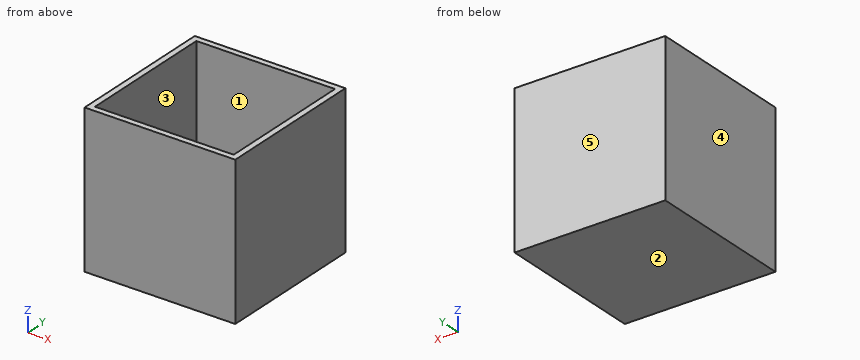
Autodesk Fusion 360 part; units mm, degrees
sketch "Sketch1" plane through (0, 0, 0) normal (0, 1, 0) x (1, 0, 0)
  line L0 (10, 10) -> (-10, 10)
  line L1 (-10, 10) -> (-10, -10)
  line L2 (-10, -10) -> (10, -10)
  line L3 (10, -10) -> (10, 10)
  line L4 (10, 10) -> (-10, -10) construction
  line L5 (-10, 10) -> (10, -10) construction
  dimension "d1" = 20
  dimension "d2" = 20
extrude "Extrude1" add sketch "Sketch1" along normal blind 20
sketch "Sketch2" plane through (0, 0, 10) normal (0, 0, 1) x (-1, 0, 0)
  line L0 (10, 0) -> (-10, 0)
  line L1 (-10, 0) -> (-10, -20)
  line L2 (-10, -20) -> (10, -20)
  line L3 (10, -20) -> (10, 0)
  line L4 (9.2, -0.8) -> (9.2, -19.2)
  line L5 (9.2, -19.2) -> (-9.2, -19.2)
  line L6 (-9.2, -19.2) -> (-9.2, -0.8)
  line L7 (-9.2, -0.8) -> (9.2, -0.8)
  dimension "d5" = 0.8
  dimension "d6" = 0.8
  dimension "d7" = 0.8
  dimension "d8" = 0.8
extrude "Extrude2" cut sketch "Sketch2" against normal blind 19.2 contours L4 L5 L6 L7
The model under review builds one solid part; all positions refer to its coordinate system, in mm. Face numbers are marked on the shaded views. A direction names the side the tool comes from. Give positions to 0.01 mm unless a question says otherwise; leave off trailing zeros. Write each loop counter-clockwise with the first axis right and the second up, starting at its lowest first coordinate (ties: lowest second). Pieces come first, ordered by that corner, then holes. Notation, with made-up numbers: M 22.5,-31 L 61.5,-31 A4 ccw 61.5,-25 Z; hole C -15.5,5 d2. An arc over 180 degrees is marked long. One line per question, with ' | ' between items. Start each with the question number.
Item 1: We need section C-C on y = 3. Write out the cut boundary in (x, z).
Item 2: We need section A-A on z = 3.5. Write out the cut boundary in (x, y), plus the area to 3 significant figures.
Item 3: Draft analysis for pull direction X (two halves, no side actions). For the marked faces 3, 4 and 5, state which applies: released by +X, released by -X, zero draft, split by the parting line, or undercut.
Item 4: For the marked faces 1 and 2, list the 3-axis set-ups (+Z, -Z, +X, -X, +Y, -Y) from which the entire face can be reached by the end or side of a thin tool; tool diameter is ignored.
Item 5: For pin 1 (9 mm diameter, centred on x = -3.5, y = 6.5, fed in from +Z), flat-tipped, find the tip position at first contact; note if it passes through.
Item 6: Wall thickness on line 1 (X direction, y = 2, z = -8.5); line 2 (Y direction, x = 7.75, z = 7.5); line 3 (Z direction, x = 7, y = 18): over which ranges is each line inside the solid? List them lowest first. Write a range as from..to.
Item 7: We need section B-B on x = 3. Write out the cut boundary in (y, z).
Results found:
1) outline: M -10,-10 L 10,-10 L 10,10 L 9.2,10 L 9.2,-9.2 L -9.2,-9.2 L -9.2,10 L -10,10 Z
2) outline: M -10,0 L 10,0 L 10,20 L -10,20 Z; hole M -9.2,0.8 L 9.2,0.8 L 9.2,19.2 L -9.2,19.2 Z | area: 61.4 mm2
3) face 3: undercut | face 4: released by -X | face 5: zero draft
4) face 1: +Z | face 2: -Z, +X, -X, +Y, -Y
5) pin 1: stops at z = -9.2
6) line 1: x = -10..-9.2, 9.2..10 | line 2: y = 0..0.8, 19.2..20 | line 3: z = -10..-9.2
7) outline: M 0,-10 L 20,-10 L 20,10 L 19.2,10 L 19.2,-9.2 L 0.8,-9.2 L 0.8,10 L 0,10 Z
